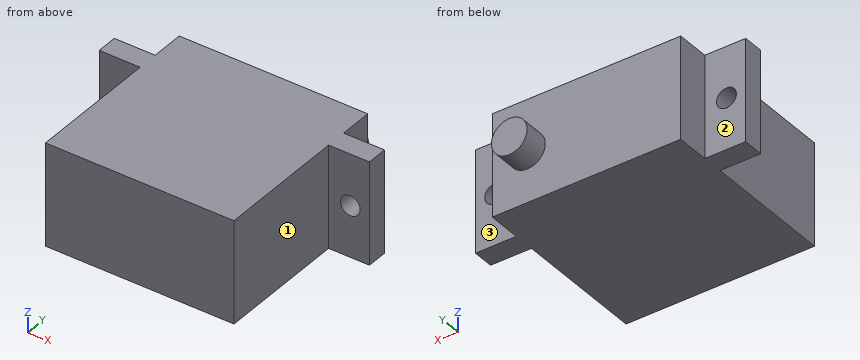
Autodesk Inventor part; units mm, degrees
ref_plane "YZ Plane" through (0, 0, 0) normal (1, 0, 0) x (0, 1, 0)
ref_plane "XZ Plane" through (0, 0, 0) normal (0, 1, 0) x (-1, 0, 0)
ref_plane "XY Plane" through (0, 0, 0) normal (0, 0, 1) x (1, 0, 0)
sketch "Sketch1" plane through (0, 0, 0) normal (0, 0, 1) x (1, 0, 0)
  line L0 (-11.25, 0) -> (11.25, 0)
  line L1 (11.25, 0) -> (11.25, 15.72)
  line L2 (11.25, 15.72) -> (16.13, 15.72)
  line L3 (16.13, 15.72) -> (16.13, 18.22)
  line L4 (16.13, 18.22) -> (11.25, 18.22)
  line L5 (11.25, 18.22) -> (11.25, 22.22)
  line L6 (11.25, 22.22) -> (-11.25, 22.22)
  line L7 (-11.25, 22.22) -> (-11.25, 18.22)
  line L8 (-11.25, 18.22) -> (-16.13, 18.22)
  line L9 (-16.13, 18.22) -> (-16.13, 15.72)
  line L10 (-16.13, 15.72) -> (-11.25, 15.72)
  line L11 (-11.25, 0) -> (-11.25, 15.72)
  point P0 (0, 0)
  point P1 (0, 0)
  dimension "d0" = 22.5
  dimension "d1" = 15.72
  dimension "d2" = 4.88
  dimension "d3" = 2.5
  dimension "d4" = 4
  dimension "d5" = 4.88
extrude "Extrusion1" add sketch "Sketch1" along normal mid plane 12.23
sketch "Sketch2" plane through (-16.13, 18.22, 6.115) normal (0, 1, 0) x (1, 0, 0)
  line L0 (4.88, 12.23) -> (4.88, 0)
  line L1 (27.38, 0) -> (4.88, 0)
  line L2 (27.38, 12.23) -> (27.38, 0)
  line L3 (4.88, 12.23) -> (27.38, 12.23)
  line L4 (27.38, 0) -> (4.88, 0)
  line L5 (16.13, 0) -> (16.13, 12.23) construction
  line L6 (4.88, 6.115) -> (27.38, 6.115) construction
  circle A0 centre (2.295, 6.115) radius 1.185
  line L7 (27.38, 6.115) -> (4.88, 6.115) construction
  circle A1 centre (29.965, 6.115) radius 1.185
  point P0 (16.13, 6.115)
  dimension "d8" = 2.37
  dimension "d9" = 27.67
sketch "Sketch3" plane through (-11.25, 22.22, 6.115) normal (0, 1, 0) x (1, 0, 0)
  circle A0 centre (18.3104, 6.115) radius 2.1368
  point P0 (11.25, 6.115)
  dimension "d10" = 4.2736
extrude "Extrusion2" cut sketch "Sketch2" against normal up to next contours A0 | A1
extrude "Extrusion3" add sketch "Sketch3" along normal blind 3
sketch "Sketch4" plane through (-11.25, 0, 6.115) normal (0, -1, 0) x (1, 0, 0)
  circle A0 centre (-2.585, -6.115) radius 1.185
  circle A1 centre (25.085, -6.115) radius 1.185
  line L0 (22.5, -12.23) -> (22.5, 0)
  line L1 (0, 0) -> (22.5, 0)
  line L2 (0, 0) -> (0, -12.23)
  line L3 (22.5, -12.23) -> (0, -12.23)
  line L4 (0, -12.23) -> (0, 0)
  line L5 (0, -6.115) -> (22.5, -6.115) construction
  line L6 (11.25, 0) -> (11.25, -12.23) construction
  circle A2 centre (18.3104, -6.115) radius 2.1368
  point P0 (11.25, -6.115)
properties part number "micro_servo"
Part model, mm, in its own coordinate system. Face numbers are marked on the shaded views. A direction names the side the tool comes from. Round coordinates to 2 decimals unless told otherwise and drop trailing zeros. Write each loop counter-clockwise with the first axis right and the second up, starting at its lowest first coordinate (ties: lowest second). Pieces come first, ordered by that corner, then holes. Notation, with made-up numbers: (83, -39) -> (93, -39) arc R34 ccw to (93, -6) -> close; hole circle Ø5 at (59, -1). An arc over 180 degrees is marked (long way). Return JSON: item names as keys, results as strings. Group by question number.
Q1. Which spindle directions (+Z, -Z, +X, -X, +Y, -Y) get a long thin tool onto all of the face, cutting with end or side? Do the marked faces 1, 2 and 3. Say none if no direction does.
Q2. Pin check, flat tips, straight feed: pin 1 (4 mm diameter, centred on x = -14, z = -3, fed in from -Y); pin 2 (3.5 mm diameter, centred on y = 5, z = -0.5, fed in from +X); pin 3 (3.5 mm diameter, centred on y = 10, z = 0, fed in from -X). Stop position of each tip, or through.
Q3. Saw through at A-A on z = 0. Write the cut outline in (x, y).
Q4. Saw through at D-D on y = 20.5. Write the cut outline in (x, z) (3 decimals).
Q5. Probe L1, parallel to X at y = 16.75, z = 0; L2, parallel to Y at x = 5, z = -3.75; L3, parallel to Y at x = 12, z = -4. List the from-to ranges inside material, lowest first. Write a range as [from, to].
Q6. Saw through at B-B on z = 5. Write the cut outline in (x, y), plus the area to 3 significant figures.
Q7. Saw through at C-C on x = 2.5. Write the cut outline in (y, z) (3 decimals), plus the area to 3 significant figures.
Answer:
{
 "1": {"face 1": "+Z, -Z, +X, -Y", "face 2": "+Z, -Z, -X, +Y", "face 3": "+Z, -Z, +X, +Y"},
 "2": {"pin 1": "y = 15.72", "pin 2": "x = 11.25", "pin 3": "x = -11.25"},
 "3": {"outline": "(-16.13, 15.72) -> (-15.02, 15.72) -> (-15.02, 18.22) -> (-16.13, 18.22) -> close; (-12.65, 15.72) -> (-11.25, 15.72) -> (-11.25, 0) -> (11.25, 0) -> (11.25, 15.72) -> (12.65, 15.72) -> (12.65, 18.22) -> (11.25, 18.22) -> (11.25, 22.22) -> (9.2, 22.22) -> (9.2, 25.22) -> (4.92, 25.22) -> (4.92, 22.22) -> (-11.25, 22.22) -> (-11.25, 18.22) -> (-12.65, 18.22) -> close; (15.02, 15.72) -> (16.13, 15.72) -> (16.13, 18.22) -> (15.02, 18.22) -> close"},
 "4": {"outline": "(-11.25, -6.115) -> (11.25, -6.115) -> (11.25, 6.115) -> (-11.25, 6.115) -> close"},
 "5": {"L1": "[-16.13, -15.02], [-12.65, 12.65], [15.02, 16.13]", "L2": "[0, 22.22]", "L3": "[15.72, 18.22]"},
 "6": {"outline": "(-16.13, 15.72) -> (-11.25, 15.72) -> (-11.25, 0) -> (11.25, 0) -> (11.25, 15.72) -> (16.13, 15.72) -> (16.13, 18.22) -> (11.25, 18.22) -> (11.25, 22.22) -> (-11.25, 22.22) -> (-11.25, 18.22) -> (-16.13, 18.22) -> close", "area": "524 mm2"},
 "7": {"outline": "(0, -6.115) -> (22.22, -6.115) -> (22.22, 6.115) -> (0, 6.115) -> close", "area": "272 mm2"}
}
